Read the model definition and answer for the solid it produces. Units are mm, in the model's axes. A direction names the side the tool comes from. Coordinates: 2 decimals unless noted, no trailing zeros. Order: outer loops, then holes, each group sorted by start corner. A loop starts at its lowest first (then second) coordinate and runs counter-clockwise, first axis right, second up. Notation, with made-up numbers: (-16.5, 80) -> (13.5, 80) arc R23 ccw to (13.5, 118) -> close; hole circle Ø6 at (-10, 57). An arc over 180 degrees is marked (long way). Answer as a JSON object with one key per item and string values. Group by question number.
1) Section A-A on z = 1 is taken. Determine the outline of the cut face in (x, y).
2) A tool of negligible diameter and unlimited length cuts with its end or side. For faces 1 (the flat face through (0, 3, 0)), 2 (the flat face through (9.85, 2, 1)), 3 (the flat face through (12.85, 2, 0)), from which of +Z, -Z, +X, -X, +Y, -Y can it reach the whole face along a straight path? Write none if from no direction.
3) Section B-B on y = 1.25 is taken. Determine the outline of the cut face in (x, z).
4) Section C-C on z = 4.25 is taken. Determine the outline of the cut face in (x, y), and give its area (3 significant figures).
5) Consider L1, parallel to X at y = 0.45, z = -2.5; L2, parallel to X at y = 0.4, z = 4.5; L3, parallel to Z at x = 12, y = 2.4. Determine where each line is inside the solid, lowest interval first.
6) Determine the mould class of faces 4 (the cylindrical face through (16.359, 1.521, -5.297)), 5 (the cylindrical face through (-16.297, 1.521, -5.359)), 6 (the flat face through (0, 0, 0)), 7 (the flat face through (-12.85, 2, 0)) for opening direction X: released by +X, released by -X, zero draft, split by the parting line, or undercut.
7) Section D-D on x = 11.5 is taken. Determine the outline of the cut face in (y, z), and give its area (3 significant figures).
Autodesk Inventor part; units mm, degrees
ref_plane "YZ Plane" through (0, 0, 0) normal (1, 0, 0) x (0, 1, 0)
ref_plane "XZ Plane" through (0, 0, 0) normal (0, 1, 0) x (-1, 0, 0)
ref_plane "XY Plane" through (0, 0, 0) normal (0, 0, 1) x (1, 0, 0)
sketch "Sketch1" plane through (0, 0, 0) normal (0, 1, 0) x (-1, 0, 0)
  line L0 (17.5, 6.5) -> (-17.5, 6.5)
  line L1 (-17.5, 6.5) -> (-17.5, -6.5)
  line L2 (-17.5, -6.5) -> (17.5, -6.5)
  line L3 (17.5, -6.5) -> (17.5, 6.5)
  line L4 (17.5, 6.5) -> (-17.5, -6.5) construction
  line L5 (-17.5, 6.5) -> (17.5, -6.5) construction
  point P0 (0, 0)
  dimension "d0" = 35
  dimension "d1" = 13
extrude "Extrusion1" add sketch "Sketch1" along normal blind 3
fillet "Fillet1" radius 4 2 edges at (-17.5, 1.5, -6.5) (17.5, 1.5, -6.5)
sketch "Sketch2" plane through (0, 3, 0) normal (0, 1, 0) x (1, 0, 0)
  line L0 (13.5, 6.5) -> (-13.5, 6.5)
  arc A0 (-13.5, 6.5) -> (-17.5, 2.5) centre (-13.5, 2.5) ccw
  line L1 (-17.5, -6.5) -> (17.5, -6.5)
  line L2 (17.5, -6.5) -> (17.5, 2.5)
  line L3 (-9.85, 3.5) -> (-12.85, 3.5)
  line L4 (-12.85, 3.5) -> (-12.85, -6.5)
  line L5 (-12.85, -6.5) -> (-9.85, -6.5)
  line L6 (-9.85, -6.5) -> (-9.85, 3.5)
  line L7 (-9.85, 3.5) -> (-12.85, -6.5) construction
  line L8 (-12.85, 3.5) -> (-9.85, -6.5) construction
  line L9 (0, 6.5) -> (0, -6.5) construction
  line L10 (0, 0) -> (17.5, 0) construction
  line L11 (-11.35, 6.5) -> (-11.35, -3.5) construction
  line L12 (-12.85, -3.5) -> (-12.3536, -3.5)
  line L13 (-12.3536, -3.5) -> (-12.85, -6.5)
  line L14 (9.85, 3.5) -> (12.85, 3.5)
  line L15 (12.85, 3.5) -> (12.85, -6.5)
  line L16 (12.85, -6.5) -> (9.85, -6.5)
  line L17 (9.85, -6.5) -> (9.85, 3.5)
  line L18 (9.85, 3.5) -> (12.85, -6.5) construction
  line L19 (12.85, 3.5) -> (9.85, -6.5) construction
  line L20 (12.85, -3.5) -> (12.3536, -3.5)
  line L21 (12.3536, -3.5) -> (12.85, -6.5)
  point P0 (-11.35, -1.5)
  point P1 (13.5, 2.5)
  point P2 (11.35, -1.5)
  point P3 (11.35, -3.5)
  dimension "d6" = 9.85
  dimension "d7" = 3
  dimension "d9" = 3
  dimension "d10" = 10
  dimension "d15" = 9.396
  dimension "d16" = 10
extrude "Extrusion2" cut sketch "Sketch2" against normal up to next contours L13 L12 L4 L3 L6 L1 | L17 L14 L15 L20 L21 L1
fillet "Fillet2" radius 1 4 edges at (-12.85, 1.5, 6.5) (-9.85, 1.5, 6.5) (9.85, 1.5, 6.5) (12.85, 1.5, 6.5)
equation "\"BendRadius\" = Thickness"
equation "\"BendReliefWidth\" = Thickness"
equation "\"BendReliefDepth\" = 0.5 * Thickness"
equation "\"CornerReliefSize\" = 4 * Thickness"
equation "\"MinimumRemnant\" = 2 * Thickness"
equation "\"TransitionRadius\" = BendRadius"
equation "\"JacobiRadiusSize\" = Thickness"
equation "\"GapSize\" = Thickness"
properties part number "link" material "Glass"
Worked answers:
{
 "1": {"outline": "(-17.5, 0) -> (-12.85, 0) -> (-12.85, 3) -> (-17.5, 3) -> close; (-9.85, 0) -> (9.85, 0) -> (9.85, 3) -> (-9.85, 3) -> close; (12.85, 0) -> (17.5, 0) -> (17.5, 3) -> (12.85, 3) -> close"},
 "2": {"face 1": "+Z, -Z, +X, -X, +Y", "face 2": "+Z, +Y, -Y", "face 3": "+Y, -Y"},
 "3": {"outline": "(-17.5, -2.5) arc R4 ccw to (-13.5, -6.5) -> (13.5, -6.5) arc R4 ccw to (17.5, -2.5) -> (17.5, 6.5) -> (13.7, 6.5) arc R1 ccw to (12.71, 5.66) -> (12.35, 3.5) -> (12.85, 3.5) -> (12.85, -3.5) -> (9.85, -3.5) -> (9.85, 5.5) arc R1 ccw to (8.85, 6.5) -> (-8.85, 6.5) arc R1 ccw to (-9.85, 5.5) -> (-9.85, -3.5) -> (-12.85, -3.5) -> (-12.85, 3.5) -> (-12.35, 3.5) -> (-12.71, 5.66) arc R1 ccw to (-13.7, 6.5) -> (-17.5, 6.5) -> close"},
 "4": {"outline": "(-17.5, 0) -> (-12.48, 0) -> (-12.48, 3) -> (-17.5, 3) -> close; (-9.85, 0) -> (9.85, 0) -> (9.85, 3) -> (-9.85, 3) -> close; (12.48, 0) -> (17.5, 0) -> (17.5, 3) -> (12.48, 3) -> close", "area": "89.2 mm²"},
 "5": {"L1": "x = -17.5 to -12.85, -9.85 to 9.85, 12.85 to 17.5", "L2": "x = -17.5 to -12.52, -9.85 to 9.85, 12.52 to 17.5", "L3": "z = -6.5 to -3.5"},
 "6": {"face 4": "released by +X", "face 5": "released by -X", "face 6": "zero draft", "face 7": "undercut"},
 "7": {"outline": "(0, -6.5) -> (3, -6.5) -> (3, -3.5) -> (0, -3.5) -> close", "area": "9.00 mm²"}
}
